from build123d import *

# Parameters (mm, degrees)
F1_DEPTH = 9.525
F2_R     = 1.4605
F3_DEPTH = 100.331
F4_R     = 1.5875
F5_DEPTH = 9.526


with BuildPart() as f1:
    # F0 (on Top) → F1 (new body)
    with BuildSketch(Plane.XY):
        Polygon((57.15, 100.33), (57.15, 104.14), (12.7, 104.14), (12.7, 91.44), (0, 91.44), (-12.7, 91.44), (-12.7, 104.14), (-57.15, 104.14), (-57.15, 100.33), (-66.04, 100.33), (-66.04, 97.79), (-57.15, 97.79), (-57.15, 91.44), (-66.04, 91.44), (-66.04, 88.9), (-57.15, 88.9), (-57.15, 0), (0, 0), (57.15, 0), (57.15, 88.9), (66.04, 88.9), (66.04, 91.44), (57.15, 91.44), (57.15, 97.79), (66.04, 97.79), (66.04, 100.33), align=None)
    extrude(amount=F1_DEPTH)

    # F2 (on face) → F3 (cut, through all)
    with BuildSketch(Plane(origin=(0, 100.33, 0), x_dir=(-1, 0, 0), z_dir=(0, 1, 0))):
        with Locations((-61.595, 4.7625)):
            Circle(F2_R)
        with Locations((61.595, 4.7625)):
            Circle(F2_R)
    extrude(amount=-F3_DEPTH, mode=Mode.SUBTRACT)

    # F4 (on face) → F5 (cut, through all)
    with BuildSketch(Plane(origin=(0, 0, 0), x_dir=(1, 0, 0), z_dir=(0, 0, -1))):
        with Locations((50.8, -81.28)):
            Circle(F4_R)
        with Locations((50.8, -66.04)):
            Circle(F4_R)
        with Locations((-50.8, -81.28)):
            Circle(F4_R)
        with Locations((-50.8, -66.04)):
            Circle(F4_R)
    extrude(amount=-F5_DEPTH, mode=Mode.SUBTRACT)


solid = f1.part
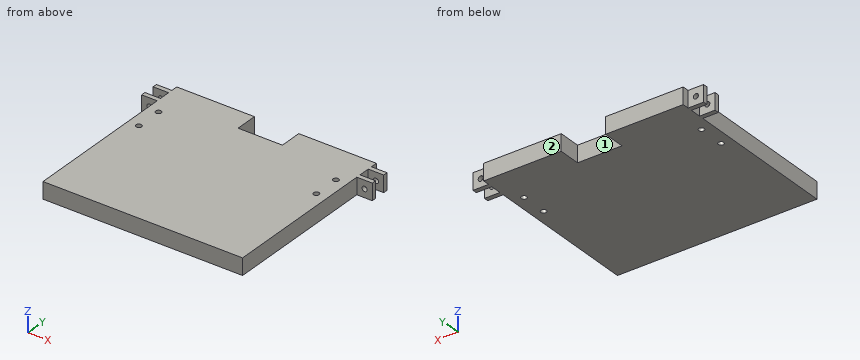
CAD build for the part. Positions are in the model's coordinates, mm. Face numbers are marked on the shaded views. Round coordinates to 2 decimals unless told otherwise and drop trailing zeros. Order: outer loops, then holes, each group sorted by start corner. A loop starts at its lowest first (then second) coordinate and runs counter-clockwise, first axis right, second up. Notation, with made-up numbers: (88, -29.5) -> (125, -29.5) arc R21 cw to (125, 5.5) -> close; hole circle Ø11 at (35.5, 26.25). An arc over 180 degrees is marked (long way). Write each question's results on one line, items separated by ' | '.
1. Pull direction X, two halves, no side cores. Call the marked faces 1 and 2: pulls with the +X half, pulls with the -X half, needs draft (parallel to the pull), parting line crosses it, or undercut.
Findings below:
face 1: undercut | face 2: needs draft
2. Cut at D-D (y = 41). Give the cut face in (x, z) (3 decimals).
Findings below:
outline: (-57.15, 0) -> (57.15, 0) -> (57.15, 9.525) -> (-57.15, 9.525) -> close
3. Cut at B-B (x = 50.8). Give the cut face in (y, z) (1 decimal).
Findings below:
outline: (0, 0) -> (64.5, 0) -> (64.5, 9.5) -> (0, 9.5) -> close; (67.6, 0) -> (79.7, 0) -> (79.7, 9.5) -> (67.6, 9.5) -> close; (82.9, 0) -> (104.1, 0) -> (104.1, 9.5) -> (82.9, 9.5) -> close
4. Wall check: line 1 along X through (y, z) = (81.28, 6.5); line 2 along Y through (x, z) = (50.8, 4.5); line 3 along Y through (x, z) = (-3.5, 9.25). Give the ranges that are in metal, low to high. Write a range as [from, to].
Findings below:
line 1: x = [-57.15, -52.39], [-49.21, 49.21], [52.39, 57.15] | line 2: y = [0, 64.45], [67.63, 79.69], [82.87, 104.14] | line 3: y = [0, 91.44]
5. Cut at A-A (y = 81.28). Count the separate pieces of the cut face and the enclosed holes in it, plus the area to 3 significant figures.
Findings below:
separate pieces: 3 | enclosed holes: 0 | area: 1,030 mm²
6. Flat gauge pins, fed straight in: P1, Ø2.5, axis at x = 61.6, z = 4.76, coming from the +Y side; P2, Ø3, axis at y = 62, z = 6.5, coming from the -X side; P3, Ø3, axis at y = 95, z = 6, coming from the +X side; P4, Ø4, axis at x = -61.6, z = 4.76, coming from the -Y side. Where does each tip first touch, or does it go through?
Findings below:
P1: passes through | P2: stops at x = -57.15 | P3: stops at x = 57.15 | P4: stops at y = 88.9
